Verification items for the finished model (mm, model axes). Face numbers are marked on the shaded views. Give positions to 0.01 mm unless a question says otherwise; leave off trailing zeros. Order: outer loops, then holes, each group sorted by start corner. A loop starts at its lowest first (then second) coordinate and runs counter-clockwise, first axis right, second up. Notation, with made-up numbers: (78, -30.5) - (86, -30.5) arc R22 cw to (86, -7.5) - close; hole circle Ø4 at (-28, 35). An arc over 180 degrees is marked (long way). Answer as a JSON object with one key per item and string values.
```python
from build123d import *

# Parameters (mm, degrees)
SKETCH1_W           = 1270
SKETCH1_H           = 1016
BOSS_EXTRUDE1_DEPTH = 1016


with BuildPart() as part:
    # Sketch1 → Boss-Extrude1 (new body)
    with BuildSketch(Plane(origin=(0, 0, 0), x_dir=(1, 0, 0), z_dir=(0, 1, 0))):
        with Locations((635, 508)):
            Rectangle(SKETCH1_W, SKETCH1_H)
    extrude(amount=BOSS_EXTRUDE1_DEPTH)

    # Sketch2 → Cut-Loft3 section 0
    with BuildSketch(Plane(origin=(0, 1016, 0), x_dir=(1, 0, 0), z_dir=(0, 1, 0)), mode=Mode.PRIVATE) as cut_loft3_s0:
        with BuildLine():
            Line((487.697722316, 0), (683.341932375, 532.014117673))
            Line((683.341932375, 532.014117673), (1270, 316.275003987))
            Line((1270, 316.275003987), (1270, 0))
            Line((1270, 0), (487.697722316, 0))
        make_face()
    loft([cut_loft3_s0.sketch, Vertex(1270, 605.056510384, 0)], mode=Mode.SUBTRACT)


solid = part.part
```
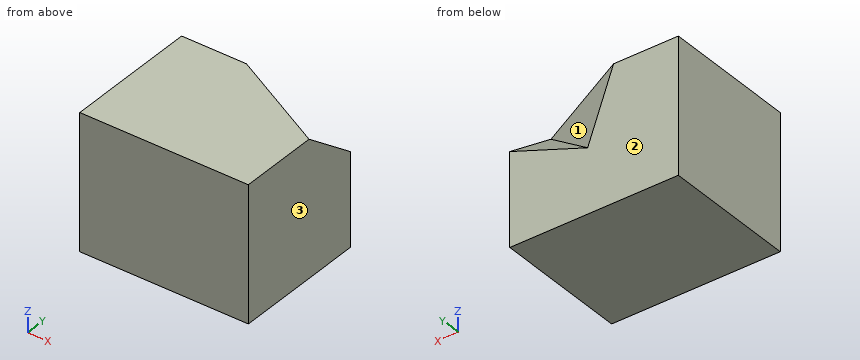
(1) Section check C-C (x = 1128). Record the cut outline in (y, z), then the cut area to 3 significant figures.
Computed values:
{"outline": "(0, -1016) - (1016, -1016) - (1016, -368.49) - (704.52, -128.77) - (679.65, 0) - (0, 0) - close", "area": "953,000 mm²"}
(2) Section check A-A (y = 841). Record the cut outline in (x, z), then the cut area to 3 significant figures.
Computed values:
{"outline": "(0, -1016) - (1270, -1016) - (1270, -181.59) - (933.17, -305.46) - (820.84, 0) - (0, 0) - close", "area": "1,190,000 mm²"}
(3) Section check B-B (z = -401). Record the cut outline in (x, y).
Computed values:
{"outline": "(0, 0) - (1270, 0) - (1270, 1016) - (1039.61, 1016) - (827.81, 914.8) - (635.16, 1016) - (0, 1016) - close"}
(4) Release check for a two-part mould opening along X. For the marked faces 1, 2 and 3 record: pulls with the +X half, pulls with the -X half, needs draft (parallel to the pull), parting line crosses it, or undercut.
Computed values:
{"face 1": "undercut", "face 2": "needs draft", "face 3": "pulls with the +X half"}
(5) Material ranges on line 1 along Y through (x, z) = (684.5, -125); line 2 along Z through (x, y) = (1154, 930.5); line 3 along Z through (x, y) = (963, 870.5), recorded low to high. Write a range as [from, to].
Computed values:
{"line 1": "y = [0, 936.77]", "line 2": "z = [-1016, -293.13]", "line 3": "z = [-1016, -317.19]"}
(6) Section check D-D (x = 651). Record the cut outline in (y, z), then the cut area to 3 significant figures.
Computed values:
{"outline": "(0, -1016) - (1016, -1016) - (1016, -444.07) - (930.22, 0) - (0, 0) - close", "area": "1,010,000 mm²"}
